```python
from build123d import *

# Parameters (mm, degrees)
CYLINDER044_R     = 1.4
CYLINDER044_DEPTH = 11
CYLINDER046_R     = 1.4
CYLINDER046_DEPTH = 11
CYLINDER047_R     = 1.4
CYLINDER047_DEPTH = 11
BOX059_W          = 15
BOX059_H          = 4.5
BOX059_DEPTH      = 4
FILLET009_R       = 0.5
PAD025_DEPTH      = 2
CHAMFER007_SIZE   = 1
CYLINDER045_R     = 1.4
CYLINDER045_DEPTH = 11


with BuildPart() as cylinder044:
    # Cylinder044 → Cylinder044 (new body)
    with BuildSketch(Plane(origin=(44.6, -3.4, -4.4), x_dir=(1, 0, 0), z_dir=(0, 0, 1))):
        Circle(CYLINDER044_R)
    extrude(amount=CYLINDER044_DEPTH)


with BuildPart() as cylinder046:
    # Cylinder046 → Cylinder046 (new body)
    with BuildSketch(Plane(origin=(30.3, -6.3, -4.4), x_dir=(1, 0, 0), z_dir=(0, 0, 1))):
        Circle(CYLINDER046_R)
    extrude(amount=CYLINDER046_DEPTH)


with BuildPart() as cylinder047:
    # Cylinder047 → Cylinder047 (new body)
    with BuildSketch(Plane(origin=(37.6, 8.5, -4.4), x_dir=(1, 0, 0), z_dir=(0, 0, 1))):
        Circle(CYLINDER047_R)
    extrude(amount=CYLINDER047_DEPTH)


with BuildPart() as fillet009:
    # Box059 → Box059 (new body)
    with BuildSketch(Plane(origin=(-7.4, -2.25, 2), x_dir=(1, 0, 0), z_dir=(0, 0, 1))):
        with Locations((7.5, 2.25)):
            Rectangle(BOX059_W, BOX059_H)
    extrude(amount=BOX059_DEPTH)

    # Fillet009
    fillet009_edges = [fillet009.edges().sort_by_distance(p)[0] for p in [
        (-7.4, 0, 2),
        (7.6, 0, 2),
        (0.1, -2.25, 2),
        (0.1, 2.25, 2),
    ]]
    fillet(fillet009_edges, radius=FILLET009_R)


with BuildPart() as chamfer007:
    # Sketch030 → Pad025 (new body)
    with BuildSketch(Plane.XY):
        with BuildLine():
            Line((-11.26, 20.5), (-11.26, 10.212751))
            Line((-11.26, 10.212751), (-13.853027, 10.212751))
            Line((-13.853027, 10.212751), (-13.853027, -10.212751))
            Line((-11.26, -10.212751), (-13.853027, -10.212751))
            Line((-11.26, -20.5), (-11.26, -10.212751))
            Line((11.48, -20.5), (-11.26, -20.5))
            Line((11.48, -7.97), (11.48, -20.5))
            Line((13, -7.97), (11.48, -7.97))
            Line((13, -11), (13, -7.97))
            Line((16, -11), (13, -11))
            ThreePointArc((24, -11), (20, -7), (16, -11))
            Line((63.2, -11), (24, -11))
            Line((63.2, 11), (63.2, -11))
            Line((63.2, 11), (24, 11))
            ThreePointArc((16, 11), (20, 7), (24, 11))
            Line((16, 11), (13, 11))
            Line((13, 11), (13, 7.97))
            Line((13, 7.97), (11.48, 7.97))
            Line((11.48, 7.97), (11.48, 20.5))
            Line((11.48, 20.5), (-11.26, 20.5))
        make_face()
    extrude(amount=PAD025_DEPTH)

    # Chamfer007
    chamfer007_edges = [chamfer007.edges().sort_by_distance(p)[0] for p in [
        (14.5, 11, 0),
        (13, 9.485, 0),
        (12.24, 7.97, 0),
        (11.48, 14.235, 0),
        (0.11, 20.5, 0),
        (-11.26, 15.356376, 0),
        (-12.556514, 10.212751, 0),
        (-13.853027, 0, 0),
        (-12.556514, -10.212751, 0),
        (-11.26, -15.356376, 0),
        (0.11, -20.5, 0),
        (11.48, -14.235, 0),
        (12.24, -7.97, 0),
        (13, -9.485, 0),
        (14.5, -11, 0),
        (20, -7, 0),
        (43.6, -11, 0),
        (63.2, 0, 0),
        (43.6, 11, 0),
        (20, 7, 0),
    ]]
    chamfer(chamfer007_edges, length=CHAMFER007_SIZE)


with BuildPart() as chamfer007_1:
    # Chamfer007 placement: moved
    add(chamfer007.part.moved(Location((0, 0, 6))))


with BuildPart() as f_04_pcbcoverbig:
    # Cylinder045 → Cylinder045 (new body)
    with BuildSketch(Plane(origin=(60.8, -3.4, -4.4), x_dir=(1, 0, 0), z_dir=(0, 0, 1))):
        Circle(CYLINDER045_R)
    extrude(amount=CYLINDER045_DEPTH)

    # Fusion047: union Cylinder044, Cylinder046, Cylinder047, Fillet009, Chamfer007
    add(cylinder044.part)
    add(cylinder046.part)
    add(cylinder047.part)
    add(fillet009.part)
    add(chamfer007_1.part)


solid = f_04_pcbcoverbig.part
```
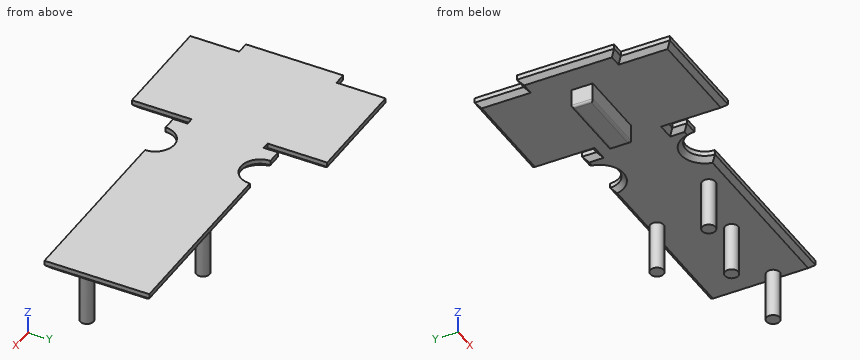
Can you work these out from the model? Positions are in its coordinate system, mm. Coordinates: 2 decimals unless noted, no trailing zeros. Order: outer loops, then holes, each group sorted by start corner. A loop starts at its lowest first (then second) coordinate and runs counter-clockwise, first axis right, second up.
1. If we section it at B-B (x = 20): Please give me the cut outline in (y, z), then the cut area to 3 significant figures.
2. If we section it at C-C (y = 13): Please give me the cut outline in (x, z), then the cut area to 3 significant figures.
3. If we section it at D-D (z = 1.25): Please give me the cut outline in (x, y), then the cut area to 3 significant figures.
4. I'm going to push flat-ended pins straight in: pin 1 (4 mm diameter, centred on y = -0.5, z = 3.5, fed in from -X); pin 2 (10 mm diameter, centred on x = 9, y = -2.5, fed in from -Z); pin 3 (1 mm diameter, centred on x = 1, z = 3.5, fed in from -Y); pin 4 (8 mm diameter, centred on x = 20, y = -12, fed in from -Z). Where does each tip first touch, or does it pass through?
5. I need wall thicknesses on line 1 (Y direction, x = 44.5, z = -1.5); line 2 (Y direction, x = 5.5, z = 3.75); line 3 (Z direction, x = 6, y = 7). Which ranges of each line are inside material? Lowest first, please.
6. If we section it at A-A (z = 4.5): Please give me the cut outline in (x, y).
Entries:
1. outline: (-7, 7) - (-6, 6) - (6, 6) - (7, 7) - (7, 8) - (-7, 8) - close
1. area: 27.0 mm2
2. outline: (-11.26, 7) - (-10.26, 6) - (10.48, 6) - (11.48, 7) - (11.48, 8) - (-11.26, 8) - close
2. area: 44.5 mm2
3. outline: circle Ø2.8 at (30.3, -6.3); circle Ø2.8 at (37.6, 8.5); circle Ø2.8 at (44.6, -3.4); circle Ø2.8 at (60.8, -3.4)
3. area: 24.6 mm2
4. pin 1: stops at x = -7.4
4. pin 2: stops at z = 2
4. pin 3: stops at y = -2.25
4. pin 4: passes through
5. line 1: y = -4.8 to -2
5. line 2: y = -2.25 to 2.25
5. line 3: z = 6 to 8
6. outline: (-7.4, -2.25) - (7.6, -2.25) - (7.6, 2.25) - (-7.4, 2.25) - close; circle Ø2.8 at (30.3, -6.3); circle Ø2.8 at (37.6, 8.5); circle Ø2.8 at (44.6, -3.4); circle Ø2.8 at (60.8, -3.4)
